CAD build for the part. Positions are in the model's coordinates, mm. A direction names the side the tool comes from. Coordinates: 2 decimals unless noted, no trailing zeros. Write each loop counter-clockwise with the first axis right and the second up, starting at its lowest first coordinate (ties: lowest second). Pieces come first, ordered by that corner, then holes. Notation, with made-up numbers: M -36,39 L 11,39 A16 ccw 11,66 Z; hole C 87.25,-19 d11. An arc over 180 degrees is marked long. Put each result on its own line as item: value. Start each with the question number.
```python
from build123d import *

# Parameters (mm, degrees)
F0_W     = 85.2193273604
F0_H     = 60.3945683688
F1_DEPTH = 127
F2_W     = 85.2193273604
F2_H     = 60.3945683688
F3_DEPTH = 25.4
F4_T     = -2.54
F5_R     = 7.5956350192
F6_DEPTH = 127


with BuildPart() as f1:
    # F0 (on Front) → F1 (new body)
    with BuildSketch(Plane.XZ):
        with Locations((3.3346693963, 1.852591522)):
            Rectangle(F0_W, F0_H)
    extrude(amount=F1_DEPTH)

    # F2 (on face) → F3 (join)
    with BuildSketch(Plane(origin=(0, 0, 0), x_dir=(-1, 0, 0), z_dir=(0, 1, 0))):
        with Locations((-3.3346693963, 1.852591522)):
            Rectangle(F2_W, F2_H)
    extrude(amount=F3_DEPTH)

    # F4
    f4_openings = [f1.faces().sort_by_distance(p)[0] for p in [
        (3.334669, 25.4, 1.852592),
    ]]
    offset(amount=F4_T, openings=f4_openings)

    # F5 (on Front) → F6 (cut, symmetric)
    with BuildSketch(Plane.XZ):
        Circle(F5_R)
    extrude(amount=F6_DEPTH, both=True, mode=Mode.SUBTRACT)


solid = f1.part
```
(1) Slice it at B-B, the plane y = -9. Write the cut outline in (x, z) (3 decimals).
(2) Two-plate mould, pull along X, no slides. Class faces 1 (the face through (4, -52, 32.05)), 2 (the face through (-6.03, -125.75, -4.62)), 3 (the face through (-39.275, -52, 1)): +X half, -X half, draft (parallel to the pull), parting line (faces both ways), or undercut.
(3) Slice it at A-A, the plane z = 0. Write the cut outline in (x, y) (3 decimals), then the cut area to 3 significant figures.
(4) Drop a flat-ended pin along its axis: pin 1 (3 mm diameter, centred on x = -22, z = 25, fed in from +Y). Give the stop position or say it passes through.
(5) Slice it at D-D, the plane z = 10. Write the cut outline in (x, y) (3 decimals), then the cut area to 3 significant figures.
(6) Drill centre lines: line 1 (X direction, y = -52.5, z = 17) (3 decimals); line 2 (Z direction, x = -3, y = -113); line 3 (Z direction, x = 0, y = -126.4). Where is each one in solid material? Low to high. Write a range as [from, to].
(7) Which spindle directions (+Z, -Z, +X, -X, +Y, -Y) get a long thin tool onto all of the face, cutting with end or side? Do faces 4 (the face through (45.944, -52, 1)), 5 (the face through (3, -124.46, 8)). Say none if no direction does.
(8) Slice it at C-C, the plane x = 0. Write the cut outline in (y, z), then the cut area to 3 significant figures.
Result set:
1. outline: M -39.275,-28.345 L 45.944,-28.345 L 45.944,32.05 L -39.275,32.05 Z; hole M -36.735,-25.805 L 43.404,-25.805 L 43.404,29.51 L -36.735,29.51 Z
2. face 1: draft
2. face 2: undercut
2. face 3: -X half
3. outline: M -39.275,-127 L -7.596,-127 L -7.596,-124.46 L -36.735,-124.46 L -36.735,25.4 L -39.275,25.4 Z; M 7.596,-127 L 45.944,-127 L 45.944,25.4 L 43.404,25.4 L 43.404,-124.46 L 7.596,-124.46 Z
3. area: 939 mm^2
4. pin 1: stops at y = -124.46
5. outline: M -39.275,-127 L 45.944,-127 L 45.944,25.4 L 43.404,25.4 L 43.404,-124.46 L -36.735,-124.46 L -36.735,25.4 L -39.275,25.4 Z
5. area: 978 mm^2
6. line 1: x = [-39.275, -36.735], [43.404, 45.944]
6. line 2: z = [-28.34, -25.8], [29.51, 32.05]
6. line 3: z = [-28.34, -7.6], [7.6, 32.05]
7. face 4: +Z, -Z, +X, +Y, -Y
7. face 5: +Y
8. outline: M -127,-28.34 L 25.4,-28.34 L 25.4,-25.8 L -124.46,-25.8 L -124.46,-7.6 L -127,-7.6 Z; M -127,7.6 L -124.46,7.6 L -124.46,29.51 L 25.4,29.51 L 25.4,32.05 L -127,32.05 Z
8. area: 876 mm^2
